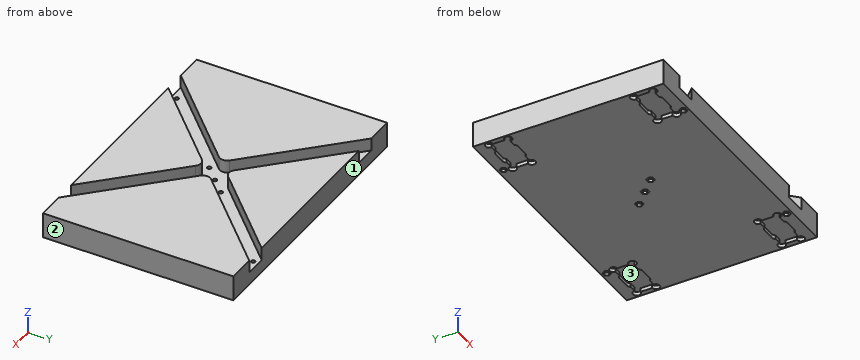
```python
from build123d import *

# Parameters (mm, degrees)
SKETCH_W        = 210
SKETCH_H        = 150
PAD_DEPTH       = 20
POCKET_DEPTH    = 10
SKETCH002_R     = 1.525
HOLE_DEPTH      = 25
POCKET001_DEPTH = 2.5
POCKET002_DEPTH = 3


with BuildPart() as part:
    # Sketch → Pad (new body)
    with BuildSketch(Plane.XY):
        Rectangle(SKETCH_W, SKETCH_H)
    extrude(amount=PAD_DEPTH)

    # Sketch001 → Pocket (cut)
    with BuildSketch(Plane.XY.offset(20)):
        with BuildLine():
            ThreePointArc((12.770342, 4.242634), (11.012983, -6e-06), (12.770342, -4.242647))
            Line((12.770342, -4.242647), (91.340443, -82.812748))
            Line((82.812735, -91.340455), (91.340443, -82.812748))
            Line((4.249755, -12.777475), (82.812735, -91.340455))
            ThreePointArc((4.249755, -12.777475), (0.007386, -11.020116), (-4.235142, -12.777091))
            Line((-4.235142, -12.777091), (-82.813511, -91.341223))
            Line((-82.813511, -91.341223), (-91.340446, -82.812743))
            Line((-12.756861, -4.243395), (-91.340446, -82.812743))
            ThreePointArc((-12.756861, -4.243395), (-10.999118, -0.00038), (-12.756847, 4.242641))
            Line((-85.748585, 77.22163), (-12.756847, 4.242641))
            Line((-85.748585, 77.22163), (-77.221622, 85.750082))
            Line((-77.221622, 85.750082), (-4.23552, 12.776728))
            ThreePointArc((-4.23552, 12.776728), (0.007012, 11.019739), (4.249391, 12.777099))
            Line((77.221622, 85.74933), (4.249391, 12.777099))
            Line((85.74933, 77.221622), (77.221622, 85.74933))
            Line((85.74933, 77.221622), (12.770342, 4.242634))
        make_face()
    extrude(amount=-POCKET_DEPTH, mode=Mode.SUBTRACT)

    # Sketch002 → Hole (cut)
    with BuildSketch(Plane.XY.offset(20)):
        with Locations((70.710678, 70.710678)):
            Circle(SKETCH002_R)
        with Locations((-70.710678, 70.710678)):
            Circle(SKETCH002_R)
        with Locations((70.710678, -70.710678)):
            Circle(SKETCH002_R)
        with Locations((-70.710678, -70.710678)):
            Circle(SKETCH002_R)
        Circle(SKETCH002_R)
        with Locations((10.606602, 10.606602)):
            Circle(SKETCH002_R)
        with Locations((-10.606602, -10.606602)):
            Circle(SKETCH002_R)
    extrude(amount=-HOLE_DEPTH, mode=Mode.SUBTRACT)

    # Sketch003 → Pocket001 (cut)
    with BuildSketch(Plane.XY):
        Polygon((69.1807, 73.360678), (67.650722, 70.710678), (69.1807, 68.060678), (72.240656, 68.060678), (73.770635, 70.710678), (72.240656, 73.360678), align=None)
        Polygon((13.666558, 10.606602), (12.13658, 13.256602), (9.076624, 13.256602), (7.546645, 10.606602), (9.076624, 7.956602), (12.13658, 7.956602), align=None)
        Polygon((3.059956, 0), (1.529978, 2.65), (-1.529978, 2.65), (-3.059956, 0), (-1.529978, -2.65), (1.529978, -2.65), align=None)
        Polygon((-7.546645, -10.606602), (-9.076624, -7.956602), (-12.13658, -7.956602), (-13.666558, -10.606602), (-12.13658, -13.256602), (-9.076624, -13.256602), align=None)
        Polygon((-72.240656, -68.060678), (-73.770635, -70.710678), (-72.240656, -73.360678), (-69.1807, -73.360678), (-67.650722, -70.710678), (-69.1807, -68.060678), align=None)
        Polygon((-67.650722, 70.710678), (-69.1807, 73.360678), (-72.240656, 73.360678), (-73.770635, 70.710678), (-72.240656, 68.060678), (-69.1807, 68.060678), align=None)
        Polygon((73.770635, -70.710678), (72.240656, -68.060678), (69.1807, -68.060678), (67.650722, -70.710678), (69.1807, -73.360678), (72.240656, -73.360678), align=None)
    extrude(amount=POCKET001_DEPTH, mode=Mode.SUBTRACT)

    # Sketch004 → Pocket002 (cut)
    with BuildSketch(Plane.XY):
        with BuildLine():
            Line((-72, -49.5), (-77.401924, -49.5))
            ThreePointArc((-77.401924, -49.5), (-78.5, -48.401924), (-80, -48))
            Line((-80, -48), (-90, -48))
            ThreePointArc((-90, -48), (-91.5, -48.401924), (-92.598076, -49.5))
            Line((-92.598076, -49.5), (-98, -49.5))
            ThreePointArc((-98, -49.5), (-103.12132, -47.37868), (-101, -52.5))
            Line((-101, -52.5), (-101, -61.5))
            ThreePointArc((-101, -61.5), (-103.12132, -66.62132), (-98, -64.5))
            Line((-98, -64.5), (-92.598076, -64.5))
            ThreePointArc((-92.598076, -64.5), (-91.5, -65.598076), (-90, -66))
            Line((-90, -66), (-80, -66))
            ThreePointArc((-80, -66), (-78.5, -65.598076), (-77.401924, -64.5))
            Line((-77.401924, -64.5), (-72, -64.5))
            ThreePointArc((-72, -64.5), (-66.87868, -66.62132), (-69, -61.5))
            Line((-69, -61.5), (-69, -52.5))
            ThreePointArc((-69, -52.5), (-66.87868, -47.37868), (-72, -49.5))
        make_face()
        with BuildLine():
            Line((72, -49.5), (77.401924, -49.5))
            ThreePointArc((80, -48), (78.5, -48.401924), (77.401924, -49.5))
            Line((80, -48), (90, -48))
            ThreePointArc((92.598076, -49.5), (91.5, -48.401924), (90, -48))
            Line((92.598076, -49.5), (98, -49.5))
            ThreePointArc((101, -52.5), (103.12132, -47.37868), (98, -49.5))
            Line((101, -52.5), (101, -61.5))
            ThreePointArc((98, -64.5), (103.12132, -66.62132), (101, -61.5))
            Line((98, -64.5), (92.598076, -64.5))
            ThreePointArc((90, -66), (91.5, -65.598076), (92.598076, -64.5))
            Line((90, -66), (80, -66))
            ThreePointArc((77.401924, -64.5), (78.5, -65.598076), (80, -66))
            Line((77.401924, -64.5), (72, -64.5))
            ThreePointArc((69, -61.5), (66.87868, -66.62132), (72, -64.5))
            Line((69, -61.5), (69, -52.5))
            ThreePointArc((72, -49.5), (66.87868, -47.37868), (69, -52.5))
        make_face()
        with BuildLine():
            Line((-72, 49.5), (-77.401924, 49.5))
            ThreePointArc((-80, 48), (-78.5, 48.401924), (-77.401924, 49.5))
            Line((-80, 48), (-90, 48))
            ThreePointArc((-92.598076, 49.5), (-91.5, 48.401924), (-90, 48))
            Line((-92.598076, 49.5), (-98, 49.5))
            ThreePointArc((-101, 52.5), (-103.12132, 47.37868), (-98, 49.5))
            Line((-101, 52.5), (-101, 61.5))
            ThreePointArc((-98, 64.5), (-103.12132, 66.62132), (-101, 61.5))
            Line((-98, 64.5), (-92.598076, 64.5))
            ThreePointArc((-90, 66), (-91.5, 65.598076), (-92.598076, 64.5))
            Line((-90, 66), (-80, 66))
            ThreePointArc((-77.401924, 64.5), (-78.5, 65.598076), (-80, 66))
            Line((-77.401924, 64.5), (-72, 64.5))
            ThreePointArc((-69, 61.5), (-66.87868, 66.62132), (-72, 64.5))
            Line((-69, 61.5), (-69, 52.5))
            ThreePointArc((-72, 49.5), (-66.87868, 47.37868), (-69, 52.5))
        make_face()
        with BuildLine():
            Line((72, 49.5), (77.401924, 49.5))
            ThreePointArc((77.401924, 49.5), (78.5, 48.401924), (80, 48))
            Line((80, 48), (90, 48))
            ThreePointArc((90, 48), (91.5, 48.401924), (92.598076, 49.5))
            Line((92.598076, 49.5), (98, 49.5))
            ThreePointArc((98, 49.5), (103.12132, 47.37868), (101, 52.5))
            Line((101, 52.5), (101, 61.5))
            ThreePointArc((101, 61.5), (103.12132, 66.62132), (98, 64.5))
            Line((98, 64.5), (92.598076, 64.5))
            ThreePointArc((92.598076, 64.5), (91.5, 65.598076), (90, 66))
            Line((90, 66), (80, 66))
            ThreePointArc((80, 66), (78.5, 65.598076), (77.401924, 64.5))
            Line((77.401924, 64.5), (72, 64.5))
            ThreePointArc((72, 64.5), (66.87868, 66.62132), (69, 61.5))
            Line((69, 61.5), (69, 52.5))
            ThreePointArc((69, 52.5), (66.87868, 47.37868), (72, 49.5))
        make_face()
    extrude(amount=POCKET002_DEPTH, mode=Mode.SUBTRACT)


solid = part.part
```
Can you work these out from the model? Positions are in its coordinate system, mm. Face numbers are marked on the shaded views. Round coordinates to 2 decimals unless told otherwise and drop trailing zeros. Loops run counter-clockwise (first coordinate to the right, second up) from the corner with the lowest first, then second, coordinate; pieces in that order, holes last.
Item 1: Suppose I cut it at B-B, the plane y = 15.5. Write out the boundary of the cut face in (x, z), then the cut area to 3 significant figures.
Item 2: Suppose I cut it at A-A, the plane z = 17.5. Write out the boundary of the cut face in (x, y).
Item 3: Suppose I cut it at C-C, the plane x = 24.5. Write out the boundary of the cut face in (y, z).
Item 4: Please list where these lines run through material, in increasing order: L1, parallel to X at y = -24.5, z = 16.5; L2, parallel to X at y = 16.5, z = 18; L3, parallel to Y at x = -57.5, z = 13.5.
Item 5: Will this pin go through, and if not, where does the flat tip stop? pin 1 Ø4 at (x, y) = (10.5, 10.5) entering from -Z.
Item 6: If we mould it in two halves opening along X, with no side actions, what happens to the marked faces 1, 2 and 3? For each: +X half, -X half, draft (parallel to the pull), parting line (faces both ways), or undercut.
Reported:
1. outline: (-105, 0) - (105, 0) - (105, 20) - (24.03, 20) - (24.03, 10) - (6.97, 10) - (6.97, 20) - (-6.96, 20) - (-6.96, 10) - (-24.02, 10) - (-24.02, 20) - (-105, 20) - close
1. area: 3,860 mm2
2. outline: (-105, -75) - (-83.53, -75) - (-12.76, -4.24) arc R6 ccw to (-12.76, 4.24) - (-83.53, 75) - (-105, 75) - close; (-66.47, -75) - (66.47, -75) - (4.25, -12.78) arc R6 ccw to (-4.24, -12.78) - close; (-66.47, 75) - (-4.24, 12.78) arc R6 ccw to (4.25, 12.78) - (66.47, 75) - close; (12.77, -4.24) - (83.53, -75) - (105, -75) - (105, 75) - (83.53, 75) - (12.77, 4.24) arc R6 ccw to start
3. outline: (-75, 0) - (75, 0) - (75, 20) - (33.03, 20) - (33.03, 10) - (15.97, 10) - (15.97, 20) - (-15.97, 20) - (-15.97, 10) - (-33.03, 10) - (-33.03, 20) - (-75, 20) - close
4. L1: x = -105 to -33.02, -15.96 to 15.97, 33.03 to 105
4. L2: x = -105 to -25.02, -7.96 to 7.97, 25.03 to 105
4. L3: y = -75 to -66.03, -48.98 to 48.98, 66.03 to 75
5. pin 1: stops at z = 2.5
6. face 1: draft
6. face 2: +X half
6. face 3: undercut
